Could you check a few things on this drawing? It's one solid part, dimensions in mm from its lowest x, y, z. A direction names the side the tool comes from. Coordinates: 2 decimals unless noted, no trailing zeros. Write each loop counter-clockwise with the first axis right and the second up, starting at its lowest first coordinate (ties: lowest second). Pieces come first, ordered by that corner, then holes.
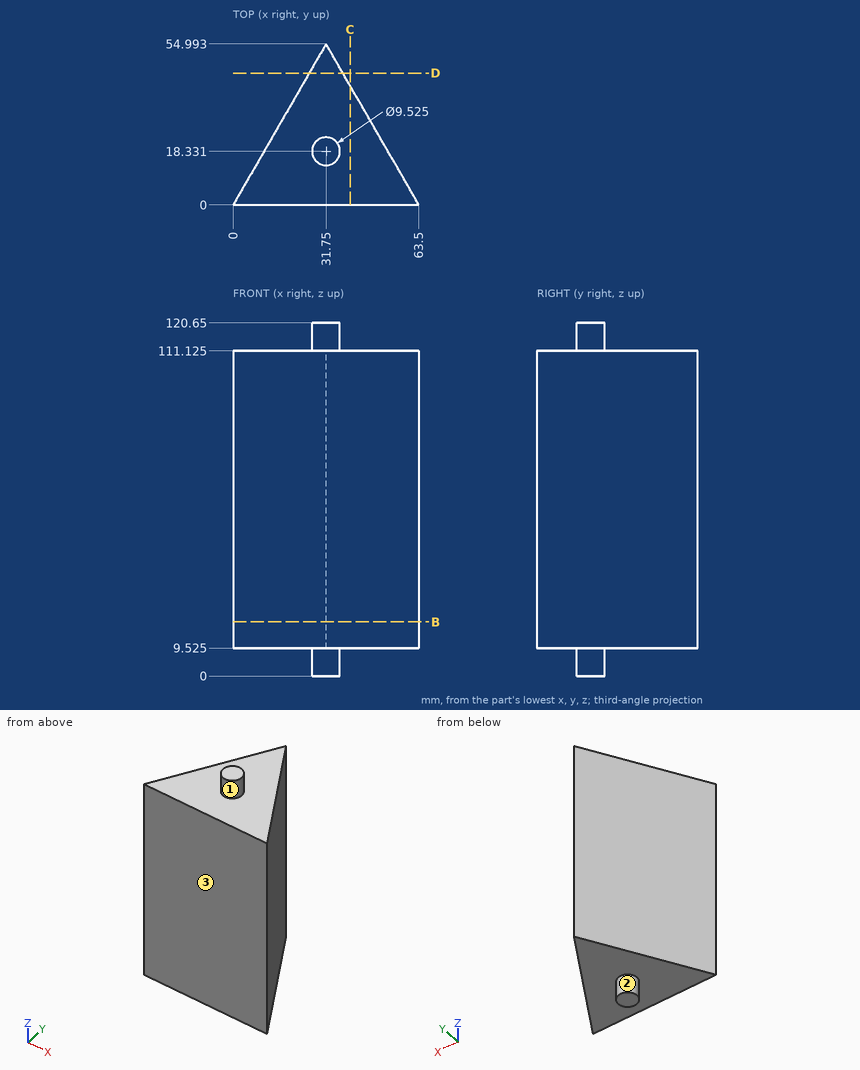
1) Will these pins go through, and if not, where does the flat tip stop? pin 1 (12 mm diameter, centred on x = 41.5, y = 23, fed in from -Z) (3 decimals); pin 2 (10 mm diameter, centred on y = 35.5, z = 54.5, fed in from -X); pin 3 (8 mm diameter, centred on x = 24, y = 40.5, fed in from +Z) (3 decimals).
Values follow:
pin 1: stops at z = 9.525
pin 2: stops at x = 17.61
pin 3: stops at z = 111.125
2) Imagine slicing it at B-B on z = 18.5. Please give me the cut outline in (x, y).
Values follow:
outline: (0, 0) - (63.5, 0) - (31.75, 54.99) - close
3) Imagine slicing it at D-D on y = 45. Please give me the cut outline in (x, z) (1 decimal).
Values follow:
outline: (26, 9.5) - (37.5, 9.5) - (37.5, 111.1) - (26, 111.1) - close
4) Imagine slicing it at C-C on x = 40. Please give me the cut outline in (y, z) (1 decimal).
Values follow:
outline: (0, 9.5) - (40.7, 9.5) - (40.7, 111.1) - (0, 111.1) - close
5) I need wall thicknesses on probe 1 along Z at (x, y) = (27.5, 40.5) (1 decimal); probe 2 along Y at (x, z) = (33.5, 80.5); probe 3 along Y at (x, z) = (45, 59) (1 decimal). Which ranges of each line are inside material? Lowest first, please.
Values follow:
probe 1: z = 9.5 to 111.1
probe 2: y = 0 to 51.96
probe 3: y = 0 to 32
6) On a 3-axis mill with a long thin cutter (end or side, diameter ignored), from which of +Z, -Z, +X, -X, +Y, -Y can I reach the whole of each face in a straight line? I mean the marked faces 1, 2 and 3. Say none if no direction works.
Values follow:
face 1: +Z
face 2: -Z
face 3: +Z, -Z, +X, -X, -Y
